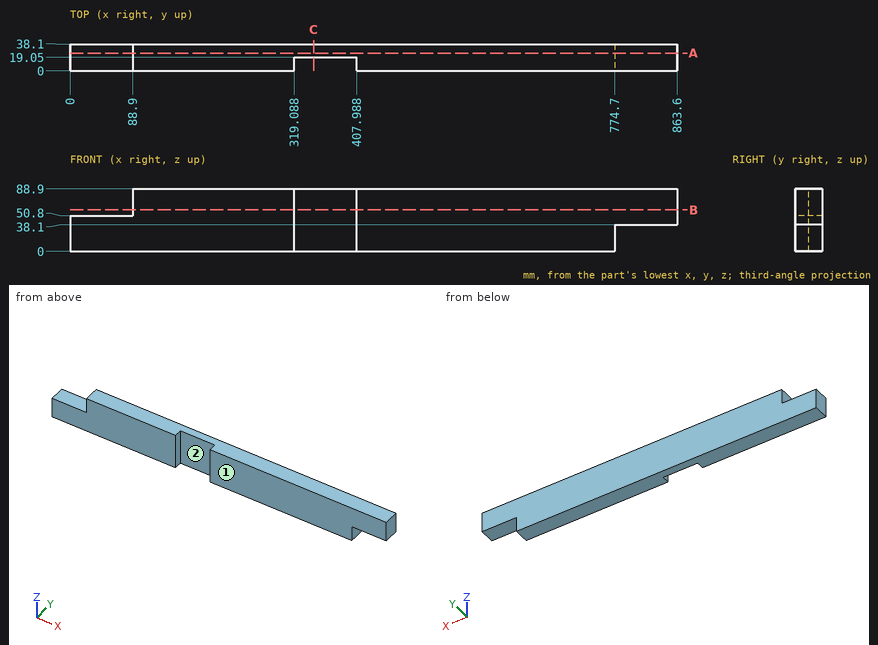
Here's the drawing with two shaded views (mm, measured from the low corner). I have some questions. Coordinates: 2 decimals unless noted, no trailing zeros. Write each loop counter-clockwise with the first axis right and the second up, starting at its lowest first coordinate (ties: lowest second). Pieces come first, ordered by that corner, then holes. Notation, with made-up numbers: (-34, -35) - (-7, -35) arc R11 cw to (-7, -20) - close; hole circle Ø1 at (-35, 6). An arc over 180 degrees is marked (long way). Return JSON: item names as keys, results as strings.
Q1. If we section it at C-C (x = 346.5): Please give me the cut outline in (y, z), then the cut area to 3 significant figures.
Computed values:
{"outline": "(19.05, 0) - (38.1, 0) - (38.1, 88.9) - (19.05, 88.9) - close", "area": "1,690 mm2"}
Q2. Please list where these lines run through material, in increasing order: L1, parallel to X at y = 2, z = 82.5; L2, parallel to X at y = 5.5, z = 15; L3, parallel to X at y = 20.5, z = 79. Write a range as from..to.
Computed values:
{"L1": "x = 88.9..319.09, 407.99..863.6", "L2": "x = 0..319.09, 407.99..774.7", "L3": "x = 88.9..863.6"}
Q3. I'm going to push flat-ended pins straight in: pin 1 Ø2 at (y, z) = (31, 18) entering from +X; pin 2 Ø11.5 at (x, y) = (64, 14.5) entering from +Z. Where does each tip first touch, or does it pass through?
Computed values:
{"pin 1": "stops at x = 774.7", "pin 2": "stops at z = 50.8"}
Q4. If we section it at B-B (z = 59): Please give me the cut outline in (x, y), then the cut area to 3 significant figures.
Computed values:
{"outline": "(88.9, 0) - (319.09, 0) - (319.09, 19.05) - (407.99, 19.05) - (407.99, 0) - (863.6, 0) - (863.6, 38.1) - (88.9, 38.1) - close", "area": "27,800 mm2"}
Q5. If we section it at A-A (y = 25): Please give me the cut outline in (x, z), then the cut area to 3 significant figures.
Computed values:
{"outline": "(0, 0) - (774.7, 0) - (774.7, 38.1) - (863.6, 38.1) - (863.6, 88.9) - (88.9, 88.9) - (88.9, 50.8) - (0, 50.8) - close", "area": "70,000 mm2"}
Q6. Thinking about a two-plate mould opening in X: for the marked faces 1 and 2, which applies, +X half, -X half, draft (parallel to the pull), parting line (faces both ways), or undercut?
Computed values:
{"face 1": "draft", "face 2": "undercut"}
